Here's how the part is built. I have some questions about the finished solid (model axes, mm). A direction names the side the tool comes from. Round coordinates to 2 decimals unless told otherwise and drop trailing zeros. Order: outer loops, then holes, each group sorted by start corner. A loop starts at its lowest first (then second) coordinate and runs counter-clockwise, first axis right, second up. Notation, with made-up numbers: (25, -37) - (63, -37) arc R18 cw to (63, -2) - close; hole circle Ø1 at (-29, -3). An arc over 180 degrees is marked (long way). Answer as a JSON object with one key per item and string values.
```python
from build123d import *

# Parameters (mm, degrees)
SKETCH1_R           = 50
BOSS_EXTRUDE1_DEPTH = 3
SKETCH2_R           = 1.5
CUT_EXTRUDE1_DEPTH  = 10
SKETCH3_W           = 14
SKETCH3_H           = 45
CUT_EXTRUDE2_DEPTH  = 10
FILLET1_R           = 1
SKETCH4_R           = 1.5
CUT_EXTRUDE3_DEPTH  = 10
FILLET2_R           = 2
CUT_EXTRUDE5_DEPTH  = 3


with BuildPart() as part:
    # Sketch1 → Boss-Extrude1 (new body)
    with BuildSketch(Plane(origin=(0, 0, 0), x_dir=(1, 0, 0), z_dir=(0, 1, 0))):
        with Locations(Location((0, 0, 0), (0, 0, 270))):
            Circle(SKETCH1_R)
    extrude(amount=BOSS_EXTRUDE1_DEPTH)

    # Sketch2 → Cut-Extrude1 (cut)
    with BuildSketch(Plane(origin=(0, 3, 0), x_dir=(1, 0, 0), z_dir=(0, 1, 0))):
        with Locations(Location((-22.75, 32.86, 0), (0, 0, 270))):
            Circle(SKETCH2_R)
        with Locations(Location((22.75, 32.86, 0), (0, 0, 270))):
            Circle(SKETCH2_R)
        with Locations(Location((22.75, 7.14, 0), (0, 0, 270))):
            Circle(SKETCH2_R)
        with Locations(Location((-22.75, 7.14, 0), (0, 0, 270))):
            Circle(SKETCH2_R)
    extrude(amount=-CUT_EXTRUDE1_DEPTH, mode=Mode.SUBTRACT)

    # Sketch3 → Cut-Extrude2 (cut)
    with BuildSketch(Plane.XZ):
        with Locations((-27, 25.5)):
            Rectangle(SKETCH3_W, SKETCH3_H)
        with Locations((27, 25.5)):
            Rectangle(SKETCH3_W, SKETCH3_H)
    extrude(amount=-CUT_EXTRUDE2_DEPTH, mode=Mode.SUBTRACT)

    # Fillet1
    fillet1_edges = [part.edges().sort_by_distance(p)[0] for p in [
        (-34, 1.5, 36.66060556),
        (-20, 1.5, 45.82575695),
        (34, 1.5, 36.66060556),
        (20, 1.5, 45.82575695),
    ]]
    fillet(fillet1_edges, radius=FILLET1_R)

    # Sketch4 → Cut-Extrude3 (cut)
    with BuildSketch(Plane.XZ):
        with Locations(Location((-40, 22.5, 0), (0, 0, 270))):
            Circle(SKETCH4_R)
        with Locations(Location((-40, -22.5, 0), (0, 0, 270))):
            Circle(SKETCH4_R)
        with Locations(Location((40, -22.5, 0), (0, 0, 270))):
            Circle(SKETCH4_R)
        with Locations(Location((40, 22.5, 0), (0, 0, 270))):
            Circle(SKETCH4_R)
    extrude(amount=-CUT_EXTRUDE3_DEPTH, mode=Mode.SUBTRACT)

    # Fillet2
    fillet2_edges = [part.edges().sort_by_distance(p)[0] for p in [
        (-34, 1.5, 3),
        (-20, 1.5, 3),
        (20, 1.5, 3),
        (34, 1.5, 3),
    ]]
    fillet(fillet2_edges, radius=FILLET2_R)

    # Sketch6 → Cut-Extrude5 (cut)
    with BuildSketch(Plane(origin=(0, 3, 0), x_dir=(1, 0, 0), z_dir=(0, 1, 0))):
        with BuildLine():
            Line((23.309994817, 27.350423227), (28.567392471, 33.519109752))
            ThreePointArc((28.567392471, 33.519109752), (29.22412311, 33.850150921), (29.920063035, 33.612346362))
            ThreePointArc((29.920063035, 33.612346362), (33.463097983, 30.086892052), (36.593306958, 26.190263189))
            ThreePointArc((36.593306958, 26.190263189), (36.756034947, 25.473044262), (36.357273652, 24.855085673))
            Line((36.357273652, 24.855085673), (29.666265874, 20.280882086))
            ThreePointArc((29.666265874, 20.280882086), (28.968053798, 20.129465624), (28.362226288, 20.508147649))
            ThreePointArc((28.362226288, 20.508147649), (26.026853987, 23.400916041), (23.397812241, 26.029644299))
            ThreePointArc((23.397812241, 26.029644299), (23.085451973, 26.672184656), (23.309994817, 27.350423227))
        make_face()
        with BuildLine():
            Line((-23.309994817, 27.350423227), (-28.567392471, 33.519109752))
            ThreePointArc((-28.567392471, 33.519109752), (-29.22412311, 33.850150921), (-29.920063035, 33.612346362))
            ThreePointArc((-29.920063035, 33.612346362), (-33.463097983, 30.086892052), (-36.593306958, 26.190263189))
            ThreePointArc((-36.593306958, 26.190263189), (-36.756034947, 25.473044262), (-36.357273652, 24.855085673))
            Line((-36.357273652, 24.855085673), (-29.666265874, 20.280882086))
            ThreePointArc((-29.666265874, 20.280882086), (-28.968053798, 20.129465624), (-28.362226288, 20.508147649))
            ThreePointArc((-28.362226288, 20.508147649), (-26.026853987, 23.400916041), (-23.397812241, 26.029644299))
            ThreePointArc((-23.397812241, 26.029644299), (-23.085451973, 26.672184656), (-23.309994817, 27.350423227))
        make_face()
    extrude(amount=-CUT_EXTRUDE5_DEPTH, mode=Mode.SUBTRACT)


solid = part.part
```
1. Imagine slicing it at D-D (y = 1.15). Give the number of separate pieces and of enclosed holes in the cut face, plus the area to 3 significant figures.
Responses:
{"separate pieces": "1", "enclosed holes": "10", "area": "6,500 mm2"}
2. For P1, Ø1.5, axis at y = 1, z = 22, coming from the +X side; P2, Ø1.5, axis at x = 36.5, y = 1.5, coming from the -Z side; P3, Ø1.5, axis at x = -29.5, y = 1, coming from the +Z side, each with a flat end and sliding along its axis, tell me the tip position at first contact or that it passes through.
Responses:
{"P1": "x = 45.26", "P2": "z = -34.96", "P3": "z = 3"}
3. Imagine slicing it at C-C (z = -22.5). List the corners of the cut face in (x, y) for me.
Responses:
{"outline": "(-44.65, 0) - (-41.5, 0) - (-41.5, 3) - (-44.65, 3) - close; (-38.5, 0) - (-32.91, 0) - (-32.91, 3) - (-38.5, 3) - close; (-26.81, 0) - (26.81, 0) - (26.81, 3) - (-26.81, 3) - close; (32.91, 0) - (38.5, 0) - (38.5, 3) - (32.91, 3) - close; (41.5, 0) - (44.65, 0) - (44.65, 3) - (41.5, 3) - close"}
4. Thinking about a two-plate mould opening in Z: for faces 1 (the face through (1.642, 1.479, -49.973)), 2 (the face through (-20, 1, 25)), 3 (the face through (33.06, 1.52, -22.6)), which applies, pulls with the +Z half, pulls with the -Z half, needs draft (parallel to the pull), parting line crosses it, or undercut?
Responses:
{"face 1": "parting line crosses it", "face 2": "needs draft", "face 3": "undercut"}
5. If I drill on L1, parallel to X at y = 1.95, z = 16; L2, parallel to X at y = 0.9, z = 12; L3, parallel to X at y = 1.55, z = 22.5, over which ranges is the centre line in solid material (lowest first)? Write a range as [from, to].
Responses:
{"L1": "[-47.37, -34], [-20, 20], [34, 47.37]", "L2": "[-48.54, -34], [-20, 20], [34, 48.54]", "L3": "[-44.65, -41.5], [-38.5, -34], [-20, 20], [34, 38.5], [41.5, 44.65]"}
6. Imagine slicing it at B-B (z = 25.5). List the corners of the cut face in (x, y) for me.
Responses:
{"outline": "(-43.01, 0) - (-34, 0) - (-34, 3) - (-43.01, 3) - close; (-20, 0) - (20, 0) - (20, 3) - (-20, 3) - close; (34, 0) - (43.01, 0) - (43.01, 3) - (34, 3) - close"}
7. Imagine slicing it at A-A (x = 40). List the corners of the cut face in (y, z) for me.
Responses:
{"outline": "(0, -30) - (3, -30) - (3, -24) - (0, -24) - close; (0, -21) - (3, -21) - (3, 21) - (0, 21) - close; (0, 24) - (3, 24) - (3, 30) - (0, 30) - close"}
8. For faces 4 (the face through (1, 3, -1)), 5 (the face through (-34, 1, 19)), 6 (the face through (33.416, 1.521, -30.139)), which set-ups out of +Z, -Z, +X, -X, +Y, -Y let a thin tool reach every point of the face, with its end or its side?
Responses:
{"face 4": "+Z, -Z, +X, -X, +Y", "face 5": "+Z, +Y, -Y", "face 6": "+Y, -Y"}
